The model under review builds one solid part; all positions refer to its coordinate system, in mm. Face numbers are marked on the shaded views. A direction names the side the tool comes from. Coordinates: 2 decimals unless noted, no trailing zeros. Order: outer loops, then holes, each group sorted by start corner. A loop starts at its lowest first (then second) coordinate and runs counter-clockwise, first axis right, second up. Notation, with made-up numbers: (54.25, -27) -> (92.25, -27) arc R33 ccw to (92.25, 11) -> close; hole circle Ø11 at (37.5, 2.5). An arc over 180 degrees is marked (long way). Put each result on its own line as item: value.
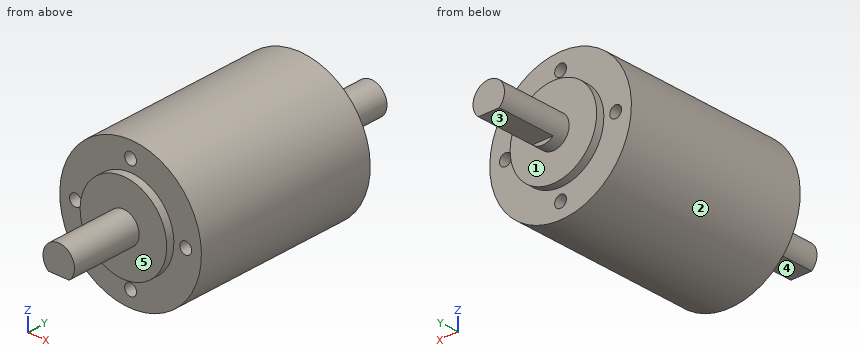
from build123d import *

# Parameters (mm, degrees)
SKETCH_1_R          = 18
EXTRUDE_1_DEPTH     = 47
SKETCH_2_R          = 11
EXTRUDE_2_DEPTH     = 2
EXTRUDE_START       = 2
SKETCH_3_R          = 11
EXTRUDE_3_DEPTH     = 2
SKETCH_4_R          = 4
EXTRUDE_4_DEPTH     = 18
EXTRUDE_START_2     = 18
SKETCH_5_R          = 4
EXTRUDE_5_DEPTH     = 18
SKETCH_6_W          = 9.252434457
SKETCH_6_H          = 4.602247191
CUT_EXTRUDE_1_DEPTH = 15
SKETCH_7_W          = 9.252434457
SKETCH_7_H          = 4.602247191
CUT_EXTRUDE_2_DEPTH = 15
SKETCH_8_R          = 1.5
CUT_EXTRUDE_3_DEPTH = 6
CUT_EXTRUDE_START   = -6
SKETCH_9_R          = 1.5
CUT_EXTRUDE_4_DEPTH = 6


with BuildPart() as part:
    # 草图1 → 凸台-拉伸1 (new body)
    with BuildSketch(Plane(origin=(0, 0, 0), x_dir=(1, 0, 0), z_dir=(0, 1, 0))):
        with Locations(Location((0, 0, 0), (0, 0, 270))):
            Circle(SKETCH_1_R)
    extrude(amount=EXTRUDE_1_DEPTH)

    # 草图2 → 凸台-拉伸2 (add)
    with BuildSketch(Plane(origin=(0, 47, 0), x_dir=(1, 0, 0), z_dir=(0, 1, 0))):
        with Locations(Location((0, 0, 0), (0, 0, 270))):
            Circle(SKETCH_2_R)
    extrude(amount=EXTRUDE_2_DEPTH)

    # 草图3 → 凸台-拉伸3 (add)
    with BuildSketch(Plane.XZ.offset(EXTRUDE_START)):
        with Locations(Location((0, 0, 0), (0, 0, 90))):
            Circle(SKETCH_3_R)
    extrude(amount=-EXTRUDE_3_DEPTH)

    # 草图4 → 凸台-拉伸4 (add)
    with BuildSketch(Plane.XZ.offset(2)):
        with Locations(Location((0, 0, 0), (0, 0, 270))):
            Circle(SKETCH_4_R)
    extrude(amount=EXTRUDE_4_DEPTH)

    # 草图5 → 凸台-拉伸5 (add)
    with BuildSketch(Plane(origin=(0, 49, 0), x_dir=(1, 0, 0), z_dir=(0, 1, 0)).offset(EXTRUDE_START_2)):
        with Locations(Location((0, 0, 0), (0, 0, 90))):
            Circle(SKETCH_5_R)
    extrude(amount=-EXTRUDE_5_DEPTH)

    # 草图6 → 切除-拉伸1 (cut)
    with BuildSketch(Plane(origin=(0, 67, 0), x_dir=(1, 0, 0), z_dir=(0, 1, 0))):
        with Locations((-0.167790263, 5.301123596)):
            Rectangle(SKETCH_6_W, SKETCH_6_H)
    extrude(amount=-CUT_EXTRUDE_1_DEPTH, mode=Mode.SUBTRACT)

    # 草图7 → 切除-拉伸2 (cut)
    with BuildSketch(Plane.XZ.offset(20)):
        with Locations((-0.167790263, -5.301123596)):
            Rectangle(SKETCH_7_W, SKETCH_7_H)
    extrude(amount=-CUT_EXTRUDE_2_DEPTH, mode=Mode.SUBTRACT)

    # 草图8 → 切除-拉伸3 (cut)
    with BuildSketch(Plane.XZ):
        with Locations(Location((0, 14, 0), (0, 0, 270))):
            Circle(SKETCH_8_R)
        with Locations(Location((14, 0, 0), (0, 0, 270))):
            Circle(SKETCH_8_R)
        with Locations(Location((0, -14, 0), (0, 0, 270))):
            Circle(SKETCH_8_R)
        with Locations(Location((-14, 0, 0), (0, 0, 270))):
            Circle(SKETCH_8_R)
    extrude(amount=-CUT_EXTRUDE_3_DEPTH, mode=Mode.SUBTRACT)

    # 草图9 → 切除-拉伸4 (cut)
    with BuildSketch(Plane(origin=(0, 47, 0), x_dir=(1, 0, 0), z_dir=(0, 1, 0)).offset(CUT_EXTRUDE_START)):
        with Locations(Location((-14, 0, 0), (0, 0, 90))):
            Circle(SKETCH_9_R)
        with Locations(Location((0, 14, 0), (0, 0, 90))):
            Circle(SKETCH_9_R)
        with Locations(Location((14, 0, 0), (0, 0, 90))):
            Circle(SKETCH_9_R)
        with Locations(Location((0, -14, 0), (0, 0, 90))):
            Circle(SKETCH_9_R)
    extrude(amount=CUT_EXTRUDE_4_DEPTH, mode=Mode.SUBTRACT)


solid = part.part
Item 1: Consider section B-B on z = -7.5. Write out the cut boundary in (x, y).
Answers below:
outline: (-16.36, 0) -> (-8.05, 0) -> (-8.05, -2) -> (8.05, -2) -> (8.05, 0) -> (16.36, 0) -> (16.36, 47) -> (8.05, 47) -> (8.05, 49) -> (-8.05, 49) -> (-8.05, 47) -> (-16.36, 47) -> close
Item 2: Consider section C-C on y = -9. Write out the cut boundary in (x, z), and give its area (3 significant figures).
Answers below:
outline: (-2.65, -3) -> (2.65, -3) arc R4 ccw (long way) to start
area: 46.6 mm^2
Item 3: For pin 1 Ø0.8 at (x, z) = (1.5, -3.5) entering from +Y; pin 2 Ø5 at (x, z) = (0, -14) entering from +Y; pin 3 Ø3 at (x, y) = (12.5, 12.5) entering from +Z, all flat-tipped, find the tip position at first contact; note any pin that passes through.
Answers below:
pin 1: y = 52
pin 2: y = 47
pin 3: z = 14.25
Item 4: For line 1 (Y direction, x = -14.5, z = 3); line 2 (Y direction, x = -5, z = 4); line 3 (X direction, y = 1.7, z = 14), list the stretches that pass through material, from the lowest coordinate up. Write a range as from..to.
Answers below:
line 1: 0..47
line 2: -2..49
line 3: -11.31..-1.5, 1.5..11.31
Item 5: Consider section A-A on x = -14. Write out the cut boundary in (y, z).
Answers below:
outline: (0, -11.31) -> (47, -11.31) -> (47, -1.5) -> (41, -1.5) -> (41, 1.5) -> (47, 1.5) -> (47, 11.31) -> (0, 11.31) -> (0, 1.5) -> (6, 1.5) -> (6, -1.5) -> (0, -1.5) -> close
Item 6: Consider section D-D on y = 24. Write out the cut boundary in (x, z), and give its area (3 significant figures).
Answers below:
outline: circle Ø36 at (0, 0)
area: 1,020 mm^2
Item 7: For the marked faces 1, 2, 3, 4 and 5, list the 3-axis set-ups (+Z, -Z, +X, -X, +Y, -Y) from which the entire face can be reached by the end or side of a thin tool; tool diameter is ignored.
Answers below:
face 1: +Y
face 2: +Y, -Y
face 3: -Z, +X, -X, +Y
face 4: -Z, +X, -X, -Y
face 5: -Y
